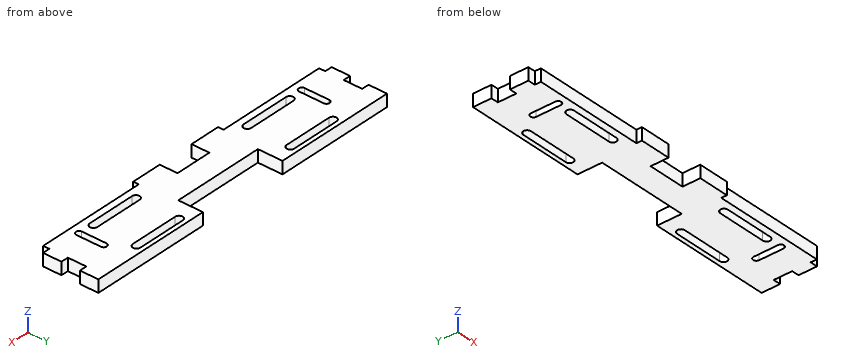
from build123d import *

# Parameters (mm, degrees)
EXTRUDE_1_DEPTH     = 10
CUT_EXTRUDE_1_DEPTH = 140.112364655
SKETCH_3_W          = 30
SKETCH_3_H          = 10
SKETCH_3_W_2        = 75
SKETCH_3_H_2        = 20
CUT_EXTRUDE_2_DEPTH = 140.112364655
SKETCH_4_W          = 25
SKETCH_4_H          = 10
EXTRUDE_2_DEPTH     = 4.5


with BuildPart() as part:
    # 草圖1 → 填料-伸長1 (new body)
    with BuildSketch(Plane.XY):
        Polygon((136, -22.5), (136, -7.5), (130, -7.5), (130, 7.5), (136, 7.5), (136, 22.5), (-136, 22.5), (-136, 7.5), (-130, 7.5), (-130, -7.5), (-136, -7.5), (-136, -22.5), (-130, -22.5), (-130, -27.5), (130, -27.5), (130, -22.5), align=None)
    extrude(amount=EXTRUDE_1_DEPTH)

    # 草圖2 → 除料-伸長1 (cut, through all)
    with BuildSketch(Plane.XY.offset(10)):
        with BuildLine():
            Line((-92.5, 19.1), (-52.5, 19.1))
            ThreePointArc((-52.5, 19.1), (-49.4, 16), (-52.5, 12.9))
            Line((-52.5, 12.9), (-92.5, 12.9))
            ThreePointArc((-92.5, 12.9), (-95.6, 16), (-92.5, 19.1))
        make_face()
        with BuildLine():
            Line((-92.5, -15.9), (-52.5, -15.9))
            ThreePointArc((-52.5, -15.9), (-49.4, -19), (-52.5, -22.1))
            Line((-52.5, -22.1), (-92.5, -22.1))
            ThreePointArc((-92.5, -22.1), (-95.6, -19), (-92.5, -15.9))
        make_face()
        with BuildLine():
            Line((52.5, 19.1), (92.5, 19.1))
            ThreePointArc((92.5, 19.1), (95.6, 16), (92.5, 12.9))
            Line((92.5, 12.9), (52.5, 12.9))
            ThreePointArc((52.5, 12.9), (49.4, 16), (52.5, 19.1))
        make_face()
        with BuildLine():
            Line((52.5, -15.9), (92.5, -15.9))
            ThreePointArc((92.5, -15.9), (95.6, -19), (92.5, -22.1))
            Line((92.5, -22.1), (52.5, -22.1))
            ThreePointArc((52.5, -22.1), (49.4, -19), (52.5, -15.9))
        make_face()
    extrude(amount=-CUT_EXTRUDE_1_DEPTH, mode=Mode.SUBTRACT)

    # 草圖3 → 除料-伸長2 (cut, through all)
    with BuildSketch(Plane.XY.offset(10)):
        with Locations((0, -22.5)):
            Rectangle(SKETCH_3_W, SKETCH_3_H)
        with Locations((0, 12.5)):
            Rectangle(SKETCH_3_W_2, SKETCH_3_H_2)
        with BuildLine():
            Line((-102.45, 0.05), (-102.45, -19.95))
            ThreePointArc((-102.45, -19.95), (-105, -22.5), (-107.55, -19.95))
            Line((-107.55, -19.95), (-107.55, 0.05))
            ThreePointArc((-107.55, 0.05), (-105, 2.6), (-102.45, 0.05))
        make_face()
        with BuildLine():
            Line((102.45, 0.05), (102.45, -19.95))
            ThreePointArc((102.45, -19.95), (105, -22.5), (107.55, -19.95))
            Line((107.55, -19.95), (107.55, 0.05))
            ThreePointArc((107.55, 0.05), (105, 2.6), (102.45, 0.05))
        make_face()
    extrude(amount=-CUT_EXTRUDE_2_DEPTH, mode=Mode.SUBTRACT)

    # 草圖4 → 填料-伸長2 (add)
    with BuildSketch(Plane.XZ.offset(27.5)):
        with Locations((-27.5, 5)):
            Rectangle(SKETCH_4_W, SKETCH_4_H)
        with Locations((27.5, 5)):
            Rectangle(SKETCH_4_W, SKETCH_4_H)
    extrude(amount=EXTRUDE_2_DEPTH)


solid = part.part
Read the model definition and answer for the solid it produces. Units are mm, in the model's axes. Give positions to 0.01 mm unless a question says otherwise; leave off trailing zeros. Write each loop counter-clockwise with the first axis right and the second up, starting at its lowest first coordinate (ties: lowest second). Pieces come first, ordered by that corner, then holes. Notation, with made-up numbers: (54.25, 39.25) - (58.25, 39.25) arc R22 cw to (58.25, 69.25) - close; hole circle Ø7 at (19, -37). An arc over 180 degrees is marked (long way). Return JSON: item names as keys, results as strings.
Q1. A cutting plane is placed at A-A, the plane x = 105. Determine the outline of the cut face in (y, z), and give its area (3 significant figures).
Reply:
{"outline": "(-27.5, 0) - (-22.5, 0) - (-22.5, 10) - (-27.5, 10) - close; (2.6, 0) - (22.5, 0) - (22.5, 10) - (2.6, 10) - close", "area": "249 mm²"}
Q2. A cutting plane is placed at B-B, the plane y = -4. Determine the outline of the cut face in (x, z), and give its area (3 significant figures).
Reply:
{"outline": "(-130, 0) - (-107.55, 0) - (-107.55, 10) - (-130, 10) - close; (-102.45, 0) - (102.45, 0) - (102.45, 10) - (-102.45, 10) - close; (107.55, 0) - (130, 0) - (130, 10) - (107.55, 10) - close", "area": "2,500 mm²"}
Q3. Given P1, Ø3, axis at x = -75, z = 4.5, coming from the -Y side; P2, Ø1.5, axis at y = -24, z = 7, coming from the -X side; P3, Ø3.5, axis at y = -29.5, z = 5.5, coming from the +X side; P4, Ø3, axis at x = 80.5, y = -19.5, coming from the +Z side, each flat-ended and moving along its own axis, determine where each tip first touches the part or whether it passes through.
Reply:
{"P1": "y = -27.5", "P2": "x = -130", "P3": "x = 40", "P4": "through"}
Q4. A cutting plane is placed at C-C, the plane y = 16. Determine the outline of the cut face in (x, z).
Reply:
{"outline": "(-136, 0) - (-95.6, 0) - (-95.6, 10) - (-136, 10) - close; (-49.4, 0) - (-37.5, 0) - (-37.5, 10) - (-49.4, 10) - close; (37.5, 0) - (49.4, 0) - (49.4, 10) - (37.5, 10) - close; (95.6, 0) - (136, 0) - (136, 10) - (95.6, 10) - close"}
Q5. Consider line 1 along Y through (x, z) = (89, 0.5); line 2 along X through (y, z) = (-9, 4.5); line 3 along X through (y, z) = (-0.5, 7). Determine where each line is inside the solid, lowest interval first. Write a range as [from, to].
Reply:
{"line 1": "[-27.5, -22.1], [-15.9, 12.9], [19.1, 22.5]", "line 2": "[-136, -107.55], [-102.45, 102.45], [107.55, 136]", "line 3": "[-130, -107.55], [-102.45, 102.45], [107.55, 130]"}
Q6. A cutting plane is placed at D-D, the plane z = 8.25. Count the separate pieces of the cut face and the enclosed holes in it, and give its area (3 significant figures).
Reply:
{"separate pieces": "1", "enclosed holes": "6", "area": "10,400 mm²"}
